```python
from build123d import *

# Parameters (mm, degrees)
SKETCH1_R                                     = 48.312804733
BOSS_EXTRUDE1_DEPTH                           = 24
CBORE_FOR_1_4_SOCKET_HEAD_CAP_SCREW1_AT_COUNT = 2
CBORE_FOR_1_4_SOCKET_HEAD_CAP_SCREW1_AT_PITCH = 25.050748534
CBORE_FOR_1_4_SOCKET_HEAD_CAP_SCREW1_2_COUNT  = 2
CBORE_FOR_1_4_SOCKET_HEAD_CAP_SCREW1_2_PITCH  = 34.539958202
CBORE_FOR_1_4_SOCKET_HEAD_CAP_SCREW1_3_COUNT  = 2
CBORE_FOR_1_4_SOCKET_HEAD_CAP_SCREW1_3_PITCH  = 34.539958202
CBORE_FOR_1_4_SOCKET_HEAD_CAP_SCREW1_4_COUNT  = 2
CBORE_FOR_1_4_SOCKET_HEAD_CAP_SCREW1_4_PITCH  = 20
CBORE_FOR_1_4_SOCKET_HEAD_CAP_SCREW1_5_COUNT  = 2
CBORE_FOR_1_4_SOCKET_HEAD_CAP_SCREW1_5_PITCH  = 25.050748534
CBORE_FOR_1_4_SOCKET_HEAD_CAP_SCREW1_6_COUNT  = 2
CBORE_FOR_1_4_SOCKET_HEAD_CAP_SCREW1_6_PITCH  = 15.698328502


with BuildPart() as part:
    # Sketch1 → Boss-Extrude1 (new body)
    with BuildSketch(Plane(origin=(0, 0, 0), x_dir=(1, 0, 0), z_dir=(0, 1, 0))):
        with Locations(Location((0, 0, 0), (0, 0, 270))):
            Circle(SKETCH1_R)
    extrude(amount=BOSS_EXTRUDE1_DEPTH)

    # Sketch3 → CBORE for 1/4 Socket Head Cap Screw1 (revolve, cut)
    with BuildSketch(Plane(origin=(0, 24, 10), x_dir=(0, 0, 1), z_dir=(1, 0, 0))):
        Polygon((0, 0), (0, 24), (3.3782, 24), (3.3782, 6.35), (5.55625, 6.35), (5.55625, 0.635), (6.19125, 0), align=None)
    cbore_for_1_4_socket_head_cap_screw1 = revolve(axis=Axis((0, 30.35, 10), (0, -1, 0)), mode=Mode.SUBTRACT)

    # CBORE for 1/4 Socket Head Cap Screw1 at: CBORE for 1/4 Socket Head Cap Screw1 ×2
    with Locations(*[Vector(-0.9862712240770178, 0, 0.16513349919874187) * (i * CBORE_FOR_1_4_SOCKET_HEAD_CAP_SCREW1_AT_PITCH) for i in range(1, CBORE_FOR_1_4_SOCKET_HEAD_CAP_SCREW1_AT_COUNT)]):
        add(cbore_for_1_4_socket_head_cap_screw1, mode=Mode.SUBTRACT)

    # CBORE for 1_4 Socket Head Cap Screw1 2: CBORE for 1/4 Socket Head Cap Screw1 ×2
    with Locations(*[Vector(-0.7153115900071431, 0, -0.6988056447979316) * (i * CBORE_FOR_1_4_SOCKET_HEAD_CAP_SCREW1_2_PITCH) for i in range(1, CBORE_FOR_1_4_SOCKET_HEAD_CAP_SCREW1_2_COUNT)]):
        add(cbore_for_1_4_socket_head_cap_screw1, mode=Mode.SUBTRACT)

    # CBORE for 1_4 Socket Head Cap Screw1 3: CBORE for 1/4 Socket Head Cap Screw1 ×2
    with Locations(*[Vector(0.7153115900071431, 0, -0.6988056447979316) * (i * CBORE_FOR_1_4_SOCKET_HEAD_CAP_SCREW1_3_PITCH) for i in range(1, CBORE_FOR_1_4_SOCKET_HEAD_CAP_SCREW1_3_COUNT)]):
        add(cbore_for_1_4_socket_head_cap_screw1, mode=Mode.SUBTRACT)

    # CBORE for 1_4 Socket Head Cap Screw1 4: CBORE for 1/4 Socket Head Cap Screw1 ×2
    with Locations(*[(0, 0, -i * CBORE_FOR_1_4_SOCKET_HEAD_CAP_SCREW1_4_PITCH) for i in range(1, CBORE_FOR_1_4_SOCKET_HEAD_CAP_SCREW1_4_COUNT)]):
        add(cbore_for_1_4_socket_head_cap_screw1, mode=Mode.SUBTRACT)

    # CBORE for 1_4 Socket Head Cap Screw1 5: CBORE for 1/4 Socket Head Cap Screw1 ×2
    with Locations(*[Vector(0.9862712240770178, 0, 0.16513349919874187) * (i * CBORE_FOR_1_4_SOCKET_HEAD_CAP_SCREW1_5_PITCH) for i in range(1, CBORE_FOR_1_4_SOCKET_HEAD_CAP_SCREW1_5_COUNT)]):
        add(cbore_for_1_4_socket_head_cap_screw1, mode=Mode.SUBTRACT)

    # CBORE for 1_4 Socket Head Cap Screw1 6: CBORE for 1/4 Socket Head Cap Screw1 ×2
    with Locations(*[Vector(-0.7644125932390737, 0, -0.6447273743975157) * (i * CBORE_FOR_1_4_SOCKET_HEAD_CAP_SCREW1_6_PITCH) for i in range(1, CBORE_FOR_1_4_SOCKET_HEAD_CAP_SCREW1_6_COUNT)]):
        add(cbore_for_1_4_socket_head_cap_screw1, mode=Mode.SUBTRACT)


solid = part.part
```
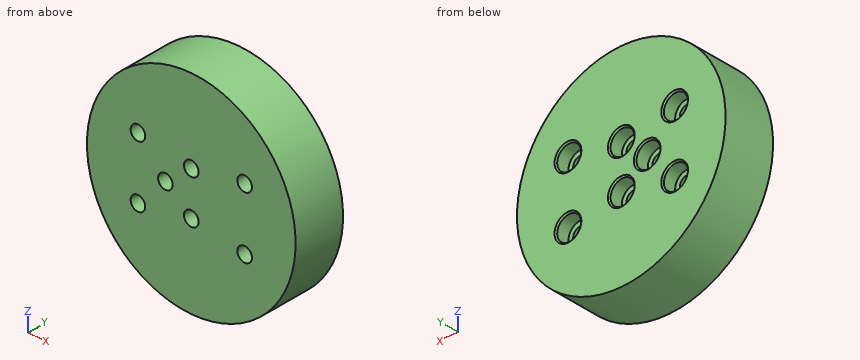
Source: CAD feature listing. Evaluate the final solid. Frame: model axes, mm. Give positions to 0.01 mm unless a question says otherwise; leave off trailing zeros. Loops run counter-clockwise (first coordinate to the right, second up) from the corner with the lowest first, then second, coordinate; pieces in that order, holes last. Notation, with made-up numbers: (71.5, 65.25) - (130.5, 65.25) arc R18 ccw to (130.5, 76.25) - close; hole circle Ø10 at (85.5, 63). An arc over 180 degrees is marked (long way). Use CSV: the item, a comma, the result in double quotes.
1) Cut plane A-A (x = 0). Output: boundary loops of the cut face in (y, z) (3 decimals), and give its area (3 significant figures).
Worked out:
outline,"(0, -48.313) - (24, -48.313) - (24, -16.191) - (23.365, -15.556) - (17.65, -15.556) - (17.65, -13.378) - (0, -13.378) - close; (0, -6.622) - (17.65, -6.622) - (17.65, -4.444) - (23.365, -4.444) - (24, -3.809) - (24, 3.809) - (23.365, 4.444) - (17.65, 4.444) - (17.65, 6.622) - (0, 6.622) - close; (0, 13.378) - (17.65, 13.378) - (17.65, 15.556) - (23.365, 15.556) - (24, 16.191) - (24, 48.313) - (0, 48.313) - close"
area,"1,940 mm^2"
2) Cut plane D-D (z = -38.5). Output: boundary loops of the cut face in (x, y), and give its area (3 significant figures).
Worked out:
outline,"(-29.19, 0) - (29.19, 0) - (29.19, 24) - (-29.19, 24) - close"
area,"1,400 mm^2"
3) Cut plane C-C (x = -12). Output: boundary loops of the cut face in (y, z) (3 decimals).
Worked out:
outline,"(0, -46.799) - (24, -46.799) - (24, -6.312) - (23.365, -5.677) - (17.65, -5.677) - (17.65, -3.499) - (0, -3.499) - close; (0, 3.257) - (17.65, 3.257) - (17.65, 5.435) - (23.365, 5.435) - (24, 6.07) - (24, 46.799) - (0, 46.799) - close"
4) Line query: line 1 (Z direction, x = 27, y = 16.25); line 2 (Z direction, x = 25.5, y = 3.5); line 3 (X direction, y = 18.5, z = -10). Output: solid intervals per line, ascending.
Worked out:
line 1,"z = -40.06 to -16.62, -11.66 to 11.66, 16.62 to 40.06"
line 2,"z = -41.04 to -17.42, -10.85 to 10.85, 17.42 to 41.04"
line 3,"x = -47.27 to -28.42, -21 to -5.56, 5.56 to 21, 28.42 to 47.27"
5) Pin query (flat end, axial travel): P1, Ø9, axis at x = 24.71, z = 14.14, coming from the +Y side; P2, Ø14.5, axis at x = -24.71, z = 14.14, coming from the -Y side; P3, Ø6, axis at x = -22, y = 4.5, coming from the +Z side; P4, Ø6.5, axis at x = 0, z = 10, coming from the +Y side. Return the tip coordinate at first contact, or that it passes through.
Worked out:
P1,"stops at y = 17.65"
P2,"stops at y = 0"
P3,"stops at z = 44.42"
P4,"passes through"
6) Cut plane B-B (y = 22). Output: boundary loops of the cut face in (x, z), and give its area (3 significant figures).
Worked out:
outline,"circle Ø96.63 at (0, 0); hole circle Ø11.11 at (-24.71, -14.14); hole circle Ø11.11 at (-24.71, 14.14); hole circle Ø11.11 at (-12, -0.12); hole circle Ø11.11 at (0, -10); hole circle Ø11.11 at (0, 10); hole circle Ø11.11 at (24.71, -14.14); hole circle Ø11.11 at (24.71, 14.14)"
area,"6,650 mm^2"
